The listing builds one solid part. Answer for the finished solid, in the listing's coordinates (mm). A direction names the side the tool comes from. Round coordinates to 2 decimals unless told otherwise and drop trailing zeros. Loops run counter-clockwise (first coordinate to the right, second up) from the corner with the lowest first, then second, coordinate; pieces in that order, holes last. Notation, with made-up numbers: (-20.5, 63) -> (-6.5, 63) arc R21 cw to (-6.5, 93) -> close; hole circle Ø6 at (76.5, 43). An arc over 180 degrees is marked (long way). One line per question, with ' | ' between items.
Autodesk Inventor part; units mm, degrees
ref_plane "YZ Plane" through (0, 0, 0) normal (1, 0, 0) x (0, 1, 0)
ref_plane "XZ Plane" through (0, 0, 0) normal (0, 1, 0) x (-1, 0, 0)
ref_plane "XY Plane" through (0, 0, 0) normal (0, 0, 1) x (1, 0, 0)
sketch "スケッチ1" plane through (0, 0, 0) normal (0, 0, 1) x (1, 0, 0)
  line L0 (-15, 0) -> (15, 0)
  line L1 (15, 0) -> (15, -26.2)
  line L2 (15, -26.2) -> (-15, -26.2)
  line L3 (-15, -26.2) -> (-15, 0)
  circle A0 centre (0, 0) radius 15
  dimension "d0" = 30
  dimension "d1" = 15
  dimension "d2" = 26.2
  dimension "d3" = 0
extrude "押し出し1" add sketch "スケッチ1" along normal blind 16
sketch "スケッチ2" plane through (0, 0, 16) normal (0, 0, 1) x (1, 0, 0)
  arc A0 (15, 0) -> (-15, 0) centre (0, 0) ccw
  line L0 (-15, -26.2) -> (-15, 0)
  line L1 (15, -26.2) -> (-15, -26.2)
  line L2 (15, 0) -> (15, -26.2)
  line L3 (-14.1, 0) -> (14.1, 0)
  line L4 (14.1, 0) -> (14.1, -25.3)
  line L5 (14.1, -25.3) -> (-14.1, -25.3)
  line L6 (-14.1, -25.3) -> (-14.1, 0)
  circle A1 centre (0, 0) radius 14.1
  dimension "d6" = 0.9
  dimension "d7" = 0.9
  dimension "d8" = 0.9
extrude "押し出し2" cut sketch "スケッチ2" against normal blind 1.5 contours A1 L3 | A1 L4 L5 L6 | L3 A1
sketch "スケッチ3" plane through (0, 0, 14.5) normal (0, 0, 1) x (1, 0, 0)
  arc A0 (14.1, 0) -> (-14.1, 0) centre (0, 0) ccw
  circle A1 centre (0, 0) radius 5.75
  dimension "d11" = 11.5
extrude "押し出し3" cut sketch "スケッチ3" against normal blind 11.7
fillet "フィレット1" radius 3 2 edges at (15, -26.2, 8) (-15, -26.2, 8)
fillet "フィレット2" radius 2.1 2 edges at (-14.1, -25.3, 15.25) (14.1, -25.3, 15.25)
sketch "スケッチ4" plane through (0, 0, 16) normal (0, 0, 1) x (1, 0, 0)
  line L0 (12, -26.2) -> (-12, -26.2)
  arc A0 (15, 0) -> (-15, 0) centre (0, 0) ccw
  line L1 (-12, -25.3) -> (12, -25.3)
  line L2 (-7.25, -25.3) -> (7.25, -25.3)
  line L3 (7.25, -25.3) -> (7.25, -26.2)
  line L4 (7.25, -26.2) -> (-7.25, -26.2)
  line L5 (-7.25, -26.2) -> (-7.25, -25.3)
  dimension "d16" = 14.5
  dimension "d17" = 7.25
extrude "押し出し4" cut sketch "スケッチ4" against normal blind 7.1
equation "\"d7\" = d6"
equation "\"d8\" = d6"
equation "\"d17\" = 0.5 * d16"
properties part number "HEDS-5500_B"
Q1. For a pull along X with two mould halves and no side action, classify faces 4 (the face through (0, -25.3, 12)), 5 (the face through (0.31, 14.097, 15.26)), 6 (the face through (14.4, -7, 16)), 7 (the face through (14.1, -25.34, 8.11)) as pulls with the +X half, pulls with the -X half, needs draft (parallel to the pull), parting line crosses it, or undercut.
Numbers:
face 4: undercut | face 5: undercut | face 6: needs draft | face 7: pulls with the +X half
Q2. A cutting plane is placed at D-D on x = 10.25. Give the vertices of the cut face in (y, z).
Numbers:
outline: (-26.2, 0) -> (10.95, 0) -> (10.95, 16) -> (9.68, 16) -> (9.68, 14.5) -> (-25.3, 14.5) -> (-25.3, 16) -> (-26.2, 16) -> close
Q3. A cutting plane is placed at C-C on x = 0. Give the vertices of the cut face in (y, z).
Numbers:
outline: (-26.2, 0) -> (15, 0) -> (15, 16) -> (14.1, 16) -> (14.1, 14.5) -> (5.75, 14.5) -> (5.75, 2.8) -> (-5.75, 2.8) -> (-5.75, 14.5) -> (-25.3, 14.5) -> (-25.3, 8.9) -> (-26.2, 8.9) -> close
Q4. Given pin 1 Ø3 at (x, z) = (2.5, 10.5) entering from +Y; pin 2 Ø1.2 at (x, z) = (8.5, 15.5) entering from +Y; pin 3 Ø8.5 at (x, y) = (1, 4) entering from +Z; pin 4 Ø2 at (x, y) = (0.5, -11) entering from -Z, each flat-ended and moving along its own axis, determine where each tip first touches the part or whether it passes through.
Numbers:
pin 1: y = 14.97 | pin 2: y = 12.75 | pin 3: z = 14.5 | pin 4: z = 0
Q5. A cutting plane is placed at A-A on z = 9.5. Give the vertices of the cut face in (x, y).
Numbers:
outline: (-15, -23.2) arc R3 ccw to (-12, -26.2) -> (-7.25, -26.2) -> (-7.25, -25.3) -> (7.25, -25.3) -> (7.25, -26.2) -> (12, -26.2) arc R3 ccw to (15, -23.2) -> (15, 0) arc R15 ccw to (-15, 0) -> close; hole circle Ø11.5 at (0, 0)
Q6. Find the intervals of material crossed by line 1 (Y direction, x = 0, z = 5.25); line 2 (Y direction, x = 0, z = 11.25); line 3 (Z direction, x = -10, y = -3), in increasing order. Write a range as from..to.
Numbers:
line 1: -26.2..-5.75, 5.75..15 | line 2: -25.3..-5.75, 5.75..15 | line 3: 0..14.5
Q7. A cutting plane is placed at B-B on y = -19.5. Give the vertices of the cut face in (x, z).
Numbers:
outline: (-15, 0) -> (15, 0) -> (15, 16) -> (14.1, 16) -> (14.1, 14.5) -> (-14.1, 14.5) -> (-14.1, 16) -> (-15, 16) -> close
Q8. For faces 1 (the face through (-7.25, -26, 12)), 2 (the face through (0, -10, 14.5)), 3 (the face through (0, 15, 8)), determine the directions among +Z, -Z, +X, -X, +Y, -Y from which every point of the face is accessible in a straight line to the end or side of a thin tool.
Numbers:
face 1: +Z, -Y | face 2: +Z | face 3: +Z, -Z, +Y
